Verification items for this drawing (mm, ordinates from the low corner). Coordinates: 2 decimals unless noted, no trailing zeros. Write each loop counter-clockwise with the first axis right and the second up, starting at its lowest first coordinate (ties: lowest second). Pieces come first, ordered by that corner, then holes.
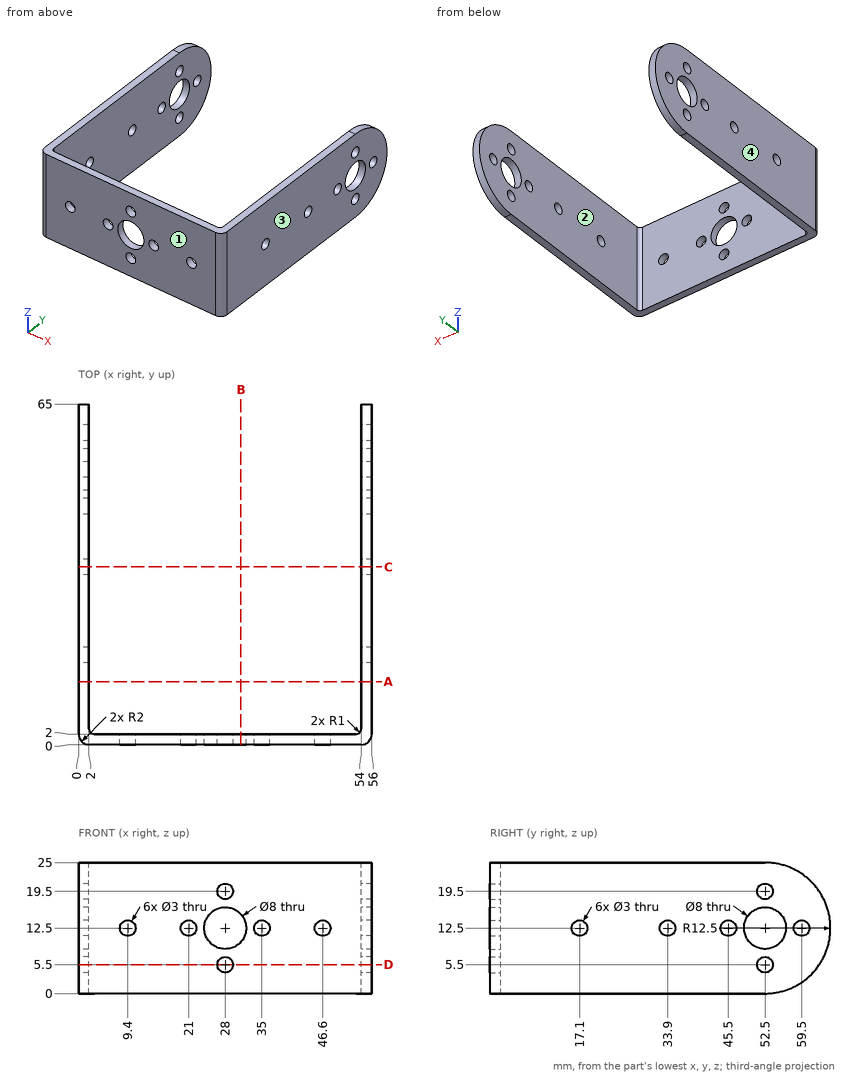
1. Sectioned sample at B-B, the plane x = 31. Record the boundary of the cut face in (y, z), and give its area (3 significant figures).
Computed values:
outline: (0, 0) - (2, 0) - (2, 9.85) - (0, 9.85) - close; (0, 15.15) - (2, 15.15) - (2, 25) - (0, 25) - close
area: 39.4 mm2
2. Sectioned sample at C-C, the plane y = 33.9. Record the boundary of the cut face in (x, z).
Computed values:
outline: (0, 0) - (2, 0) - (2, 11) - (0, 11) - close; (0, 14) - (2, 14) - (2, 25) - (0, 25) - close; (54, 0) - (56, 0) - (56, 11) - (54, 11) - close; (54, 14) - (56, 14) - (56, 25) - (54, 25) - close
3. Draft check along X on the marked faces 1, 2, 3 and 4. Enter one of: released by +X, released by -X, zero draft, split by the parting line, or undercut.
Computed values:
face 1: zero draft
face 2: undercut
face 3: released by +X
face 4: released by -X
4. Gauge pin test, flat ends, axial feed: pin 1 Ø5 at (x, z) = (35, 12.5) entering from +Y; pin 2 Ø2.5 at (y, z) = (59.5, 12.5) entering from -X. Record the tip position at first contact, or that the pin passes through.
Computed values:
pin 1: stops at y = 2
pin 2: passes through
5. Sectioned sample at D-D, the plane z = 5.5. Record the boundary of the cut face in (x, y), and give its area (3 significant figures).
Computed values:
outline: (0, 2) arc R2 ccw to (2, 0) - (26.5, 0) - (26.5, 2) - (3, 2) arc R1 cw to (2, 3) - (2, 51) - (0, 51) - close; (0, 54) - (2, 54) - (2, 62.86) - (0, 62.86) - close; (29.5, 0) - (54, 0) arc R2 ccw to (56, 2) - (56, 51) - (54, 51) - (54, 3) arc R1 cw to (53, 2) - (29.5, 2) - close; (54, 54) - (56, 54) - (56, 62.86) - (54, 62.86) - close
area: 336 mm2
6. Sectioned sample at A-A, the plane y = 12. Record the boundary of the cut face in (x, z).
Computed values:
outline: (0, 0) - (2, 0) - (2, 25) - (0, 25) - close; (54, 0) - (56, 0) - (56, 25) - (54, 25) - close
7. Thickness scan on line 1 along Z through (x, y) = (28, 1); line 2 along X through (y, z) = (56, 3); line 3 along Y through (x, z) = (0.85, 12.5). Record the ranges inside material, lowest first.
Computed values:
line 1: z = 0 to 4, 7 to 8.5, 16.5 to 18, 21 to 25
line 2: x = 0 to 2, 54 to 56
line 3: y = 0.36 to 15.6, 18.6 to 32.4, 35.4 to 44, 47 to 48.5, 56.5 to 58, 61 to 65
